Verification items for the finished model (mm, model axes). A direction names the side the tool comes from. Coordinates: 2 decimals unless noted, no trailing zeros. Order: outer loops, then holes, each group sorted by start corner. A loop starts at its lowest first (then second) coordinate and runs counter-clockwise, first axis right, second up. Notation, with made-up numbers: (-1, 63) -> (56, 63) arc R9 cw to (56, 76) -> close; hole circle Ø10 at (12.25, 33.25). An arc over 180 degrees is marked (long way). Write each question's results on one line, items separated by ' | '. Start each with the question number.
(1) Go/stop test with flat-tipped pins: pin 1 (2 mm diameter, centred on x = -10.77, y = 28.65, fed in from +Z); pin 2 (5 mm diameter, centred on x = -23.02, y = -34.54, fed in from +Z); pin 3 (1.5 mm diameter, centred on y = 31, z = 2, fed in from -X). Record where each tip stops, or that it passes through.
(2) Draft check along Y on faces 3 (the flat face through (-7.9, -21.5, 1.5)), 4 (the cylindrical face through (-34.76, -40.23, 1.48)), 5 (the cylindrical face through (-23.216, -36.023, 1.479)). Enter one of: +Y half, -Y half, draft (parallel to the pull), parting line (faces both ways), or undercut.
(3) Cross-section at C-C on x = -26. Enter the section's corners in (y, z).
(4) Cross-section at D-D on y = -31.5. Enter the section's corners in (x, z), and give its area (3 significant figures).
(5) Thickness scan on probe 1 along Y at (x, z) = (17.5, 2.25); probe 2 along Y at (x, z) = (7.5, 1.15); probe 3 along X at (y, z) = (29.5, 1.1). Record the ranges inside material, lowest first. Write a range as [from, to].
(6) Cross-section at B-B on z = 2.1. Give the number of separate pieces and of enclosed holes in the cut face, and give its area (3 significant figures).
(7) Set-up check for faces 1 (the flat face through (9.982, 30, 1)), 2 (the flat face through (20.982, 35, 1)): record each of +Z, -Z, +X, -X, +Y, -Y from which the full face is reachable in a straight line by a thin tool's end or side.
(8) Cross-section at A-A on y = -9.5. Enter the section's corners in (x, z), and give its area (3 significant figures).
Autodesk Inventor part; units mm, degrees
ref_plane "YZ Plane" through (0, 0, 0) normal (1, 0, 0) x (0, 1, 0)
ref_plane "XZ Plane" through (0, 0, 0) normal (0, 1, 0) x (-1, 0, 0)
ref_plane "XY Plane" through (0, 0, 0) normal (0, 0, 1) x (1, 0, 0)
sketch "Sketch1" plane through (0, 0, 0) normal (0, 0, 1) x (1, 0, 0)
  circle A0 centre (-10.7682, 28.6531) radius 1.7
  line L0 (-30.9487, -53.1184) -> (-37.6576, -49.0166)
  arc A1 (-38.3208, -46.2671) -> (-37.6576, -49.0166) centre (-36.6144, -47.3103) ccw
  line L1 (-38.3208, -46.2671) -> (-35.4427, -41.5596)
  arc A2 (-35.4427, -41.5596) -> (-34.2964, -38.8601) centre (-43.9745, -36.3434) ccw
  line L2 (-34.2964, -38.8601) -> (-16.5771, 29.2821)
  arc A3 (-12.739, 34.883) -> (-16.5771, 29.2821) centre (-6.899, 26.7655) ccw
  line L3 (-12.739, 34.883) -> (10.9377, 51.9167)
  arc A4 (16.7777, 53.7992) -> (10.9377, 51.9167) centre (16.7777, 43.7992) ccw
  line L4 (16.7777, 53.7992) -> (20.9818, 53.7992)
  line L5 (20.9818, 45.9992) -> (20.9818, 16.274)
  line L6 (20.9818, 16.274) -> (14.228, 11.1802)
  arc A5 (14.228, 11.1802) -> (11.8867, 8.6795) centre (20.2494, 3.1963) ccw
  line L7 (11.8867, 8.6795) -> (-28.2329, -52.5086)
  arc A6 (-4.1413, 32.6124) -> (-4.2418, 29.4427) centre (-2.9733, 30.9889) ccw
  line L8 (-4.2418, 29.4427) -> (6.7132, 20.4547)
  arc A7 (6.7132, 20.4547) -> (9.9818, 22.0009) centre (7.9818, 22.0009) ccw
  line L9 (9.9818, 22.0009) -> (9.9818, 38.8703)
  arc A8 (9.9818, 38.8703) -> (6.8138, 40.4938) centre (7.9818, 38.8703) ccw
  line L10 (6.8138, 40.4938) -> (-4.1413, 32.6124)
  circle A9 centre (17.4818, 44.7992) radius 1.2
  circle A10 centre (17.4818, 28.7992) radius 1.2
  line L11 (-16.6946, -22.1449) -> (3.4303, 8.5485)
  arc A11 (3.4303, 8.5485) -> (3.0263, 11.1914) centre (1.7578, 9.6452) ccw
  line L12 (3.0263, 11.1914) -> (-8.6289, 20.7539)
  arc A12 (-8.6289, 20.7539) -> (-11.8331, 19.711) centre (-9.8975, 19.2077) ccw
  line L13 (-11.8331, 19.711) -> (-22.01, -19.4256)
  arc A13 (-22.01, -19.4256) -> (-21.171, -21.6014) centre (-20.0743, -19.9289) ccw
  line L14 (-21.171, -21.6014) -> (-19.4638, -22.7208)
  arc A14 (-19.4638, -22.7208) -> (-16.6946, -22.1449) centre (-18.3672, -21.0482) ccw
  line L15 (20.9818, 45.9992) -> (20.9818, 53.7992)
  circle A15 centre (-31.2454, -47.0794) radius 1.5
  circle A16 centre (-23.0206, -34.5354) radius 1.5
  line L16 (-23.0206, -34.5354) -> (-31.2454, -47.0794) construction
  line L17 (-31.2454, -47.0794) -> (-33.987, -51.2608) construction
  arc A17 (-30.9487, -53.1184) -> (-28.2329, -52.5086) centre (-29.9054, -51.412) ccw
  circle A18 centre (8.5593, 12.796) radius 1.7
  line L18 (-10.7682, 28.6531) -> (8.5593, 12.796) construction
  point P0 (0, 0)
  point P1 (-30.3165, -53.5049)
  point P2 (-11.731, -27.3408)
  dimension "d2" = 3
  dimension "d3" = 3
  dimension "d5" = 2
  dimension "d6" = 5
  dimension "d7" = 15
  dimension "d8" = 3.4
  dimension "d9" = 25
extrude "Extrusion1" add sketch "Sketch1" along normal blind 3
properties part number "Tibia"
Results are:
1) pin 1: passes through | pin 2: stops at z = 3 | pin 3: stops at x = -16.27
2) face 3: -Y half | face 4: +Y half | face 5: undercut
3) outline: (-49.1, 0) -> (-6.96, 0) -> (-6.96, 3) -> (-49.1, 3) -> close
4) outline: (-32.38, 0) -> (-14.46, 0) -> (-14.46, 3) -> (-32.38, 3) -> close | area: 53.8 mm2
5) probe 1: y = [13.65, 27.6], [30, 43.6], [46, 53.8] | probe 2: y = [1.99, 11.47], [14.13, 20.06], [40.81, 49.44] | probe 3: x = [-16.52, -12.24], [-9.29, -4.31], [9.98, 16.51], [18.46, 20.98]
6) separate pieces: 1 | enclosed holes: 8 | area: 1,960 mm2
7) face 1: +Z, -Z | face 2: +Z, -Z, +X, +Y, -Y
8) outline: (-26.66, 0) -> (-19.43, 0) -> (-19.43, 3) -> (-26.66, 3) -> close; (-8.4, 0) -> (-0.03, 0) -> (-0.03, 3) -> (-8.4, 3) -> close | area: 46.8 mm2
